Build history of the part. All positions in model axes, mm. Face numbers are marked on the shaded views. A direction names the side the tool comes from. Give positions to 0.01 mm unless a question says otherwise; leave off trailing zeros. Loops run counter-clockwise (first coordinate to the right, second up) from the corner with the lowest first, then second, coordinate; pieces in that order, holes last. Notation, with made-up numbers: (51.25, 72.25) - (87.25, 72.25) arc R31 cw to (87.25, 102.25) - close; hole circle Ø6 at (78.5, 82). An arc over 180 degrees is marked (long way). Return JSON: item names as keys, results as strings. Group by question number.
1) Drop flat-ended pins along their axis: pin 1 (1 mm diameter, centred on y = 5.5, z = -8.5, fed in from -X); pin 2 (6 mm diameter, centred on y = 20.5, z = 4.5, fed in from -X); pin 3 (3 mm diameter, centred on x = 8, y = 19.5, fed in from +Z); pin 4 (1 mm diameter, centred on y = 4.5, z = 8, fed in from +X). Give the stop position or say it passes through.
2) Mould opens along Z. For the marked faces 1, 2 and 3 say: released by +Z, released by -Z, zero draft, split by the parting line, or undercut.
3) Slice it at B-B (z = 9.5). Count the separate pieces of the cut face and the enclosed holes in it, and give its area (3 significant figures).
4) 3-axis set-ups, long thin cutter, end or side, ignore diameter. For the marked faces 4, 5 and 6: which of +Z, -Z, +X, -X, +Y, -Y reach the whole face in a straight line?
5) Slice it at A-A (y = 2.75). List the corners of the cut face in (x, z).
6) Drill centre lines: probe 1 along Z at (x, y) = (-2, 6.25); probe 2 along Y at (x, z) = (-6.75, -1); probe 3 along Y at (x, z) = (5.75, -9.25). Where is each one in solid material? Low to high. Write a range as from..to.
```python
from build123d import *

# Parameters (mm, degrees)
CHANFRO1_SIZE            = 0.23
CHANFRO1_SIZE2           = 0.628371686
ESBO_O2_R                = 5
ESBO_O2_R_2              = 2.5
RESSALTO_EXTRUS_O1_DEPTH = 8


with BuildPart() as part:
    # Esboço1 → Revolução1 (revolve)
    with BuildSketch(Plane.XY, mode=Mode.PRIVATE) as revolu_o1_sk:
        Polygon((11, 0), (11, 5.894529946), (11.2, 6.01), (9.173500555, 7.18), (11.2, 8.35), (9.173500555, 9.52), (11.2, 10.69), (9.173500555, 11.86), (11.2, 13.03), (9.173500555, 14.2), (11.2, 15.37), (11.2, 16), (2.5, 16), (2.5, 0), align=None)
    revolve(revolu_o1_sk.sketch.rotate(Axis((0, 0, 0), (0, 1, 0)), 90), axis=Axis((0, 0, 0), (0, 1, 0)))

    # Chanfro1
    chanfro1_edges = [part.edges().sort_by_distance(p)[0] for p in [
        (0, 5.894529946, 11),
    ]]
    chanfro1_side = [part.faces().sort_by_distance(p)[0] for p in [
        (0, 5.952264973, 11.1),
    ]]
    chamfer(chanfro1_edges, length=CHANFRO1_SIZE, length2=CHANFRO1_SIZE2, reference=chanfro1_side[0])

    # Esboço2 → Ressalto-extrusão1 (add)
    with BuildSketch(Plane(origin=(0, 16, 0), x_dir=(1, 0, 0), z_dir=(0, 1, 0))):
        with Locations(Location((0, 0, 0), (0, 0, 270))):
            Circle(ESBO_O2_R)
        with Locations(Location((0, 0, 0), (0, 0, 90))):
            Circle(ESBO_O2_R_2, mode=Mode.SUBTRACT)
    extrude(amount=RESSALTO_EXTRUS_O1_DEPTH)


solid = part.part
```
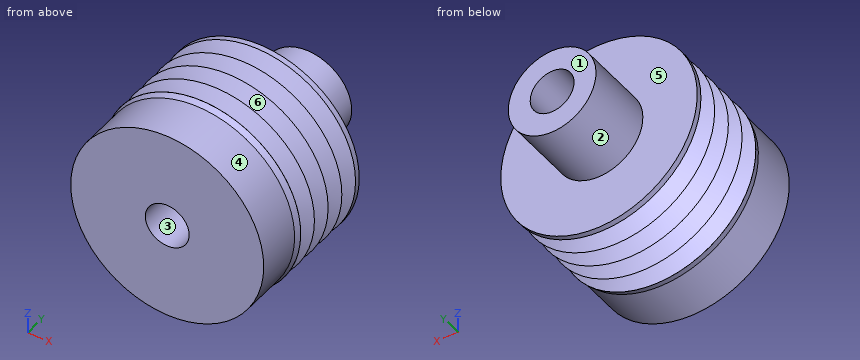
Results:
{
 "1": {"pin 1": "x = -7.68", "pin 2": "x = -4.77", "pin 3": "through", "pin 4": "x = 8.05"},
 "2": {"face 1": "zero draft", "face 2": "split by the parting line", "face 3": "undercut"},
 "3": {"separate pieces": "5", "enclosed holes": "0", "area": "135 mm2"},
 "4": {"face 4": "-Y", "face 5": "+Y", "face 6": "none"},
 "5": {"outline": "circle Ø22 at (0, 0); hole circle Ø5 at (0, 0)"},
 "6": {"probe 1": "-10.6..-1.5, 1.5..10.6", "probe 2": "0..16", "probe 3": "0..6.19, 8.17..8.53, 10.51..10.87, 12.85..13.21, 15.19..16"}
}
